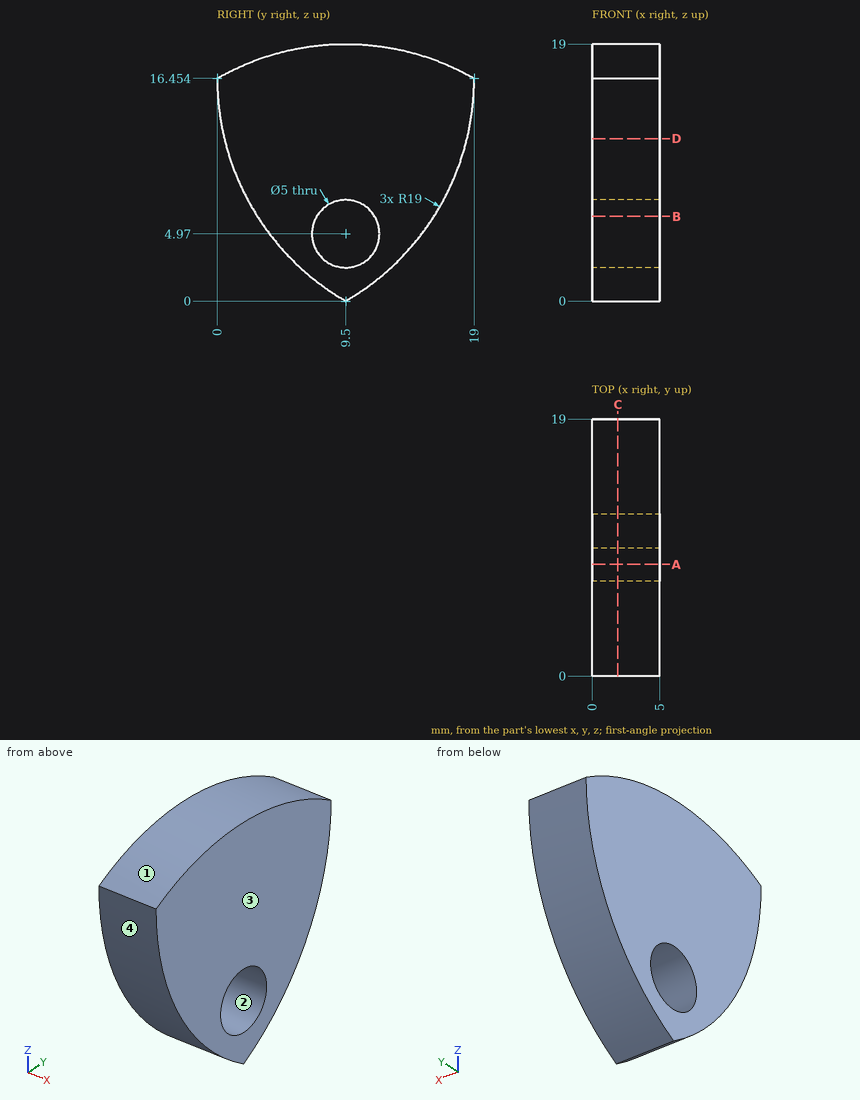
Part print with two shaded views. Sizes in mm from the minimum x, y, z corner. Round coordinates to 2 decimals unless told otherwise and drop trailing zeros. Order: outer loops, then holes, each group sorted by start corner. A loop starts at its lowest first (then second) coordinate and runs counter-clockwise, first axis right, second up. Notation, with made-up numbers: (74.5, 21) - (87.5, 21) arc R21 ccw to (87.5, 39) - close; hole circle Ø3 at (43, 44.25). An arc over 180 degrees is marked (long way). Answer as CSV lines item,"result". Start each with the question number.
1. Pin check, flat tips, straight feed: pin 1 (1 mm diameter, centred on x = 2.5, z = 15.5, fed in from +Y) (1 decimal); pin 2 (3 mm diameter, centred on x = 4.5, z = 12.5, fed in from +Y); pin 3 (1 mm diameter, centred on y = 17, z = 10.5, fed in from -X). Stop position of each tip, or through.
2. Pull direction Z, two halves, no side cores. Call the marked faces 1, 2, 3 and 4: +Z half, -Z half, draft (parallel to the pull), parting line (faces both ways), or undercut.
3. Saw through at B-B, the plane z = 6.25. Write the cut outline in (x, y), and give its area (3 significant figures).
4. Saw through at C-C, the plane x = 1.9. Write the cut outline in (y, z) (1 decimal), and give its area (3 significant figures).
5. Drill centre lines: L1, parallel to Z at x = 0.35, y = 11 (1 decimal); L2, parallel to Y at x = 2.4, z = 6.75 (1 decimal); L3, parallel to Y at x = 1.95, z = 7 (1 decimal). Where is each one in solid material? Low to high. Write a range as [from, to].
6. Saw through at A-A, the plane y = 8.25. Write the cut outline in (x, z) (1 decimal).
7. Saw through at D-D, the plane z = 12. Write the cut outline in (x, y).
Model answer:
1,pin 1,"stops at y = 19"
1,pin 2,"stops at y = 18.84"
1,pin 3,"stops at x = 0"
2,face 1,"+Z half"
2,face 2,"undercut"
2,face 3,"draft"
2,face 4,"-Z half"
3,outline,"(0, 2.97) - (5, 2.97) - (5, 7.35) - (0, 7.35) - close; (0, 11.65) - (5, 11.65) - (5, 16.03) - (0, 16.03) - close"
3,area,"43.8 mm²"
4,outline,"(0, 16.5) arc R19 ccw to (9.5, 0) arc R19 ccw to (19, 16.5) arc R19 ccw to start; hole circle Ø5 at (9.5, 5)"
4,area,"235 mm²"
5,L1,"z = [1, 3], [7, 18.9]"
5,L2,"y = [2.7, 7.7], [11.3, 16.3]"
5,L3,"y = [2.5, 8], [11, 16.5]"
6,outline,"(0, 0.8) - (5, 0.8) - (5, 2.8) - (0, 2.8) - close; (0, 7.1) - (5, 7.1) - (5, 19) - (0, 19) - close"
7,outline,"(0, 0.53) - (5, 0.53) - (5, 18.47) - (0, 18.47) - close"
